Design review of the part built by this model. Coordinates are the model's own, in mm. Give positions to 0.01 mm unless a question says otherwise; leave off trailing zeros. Order: outer loops, then holes, each group sorted by start corner. A loop starts at its lowest first (then second) coordinate and runs counter-clockwise, first axis right, second up. Notation, with made-up numbers: (40, 6) -> (68, 6) arc R34 ccw to (68, 36) -> close; hole circle Ø5 at (74, 82.5). An arc over 180 degrees is marked (long way). Return JSON: item names as keys, results as strings.
```python
from build123d import *

# Parameters (mm, degrees)
SKETCH1_W           = 93
SKETCH1_H           = 102.7
BOSS_EXTRUDE2_DEPTH = 6
SKETCH3_W           = 35
SKETCH3_H           = 100
BOSS_EXTRUDE3_DEPTH = 2.5
SKETCH4_W           = 8.5
SKETCH4_H           = 15
BOSS_EXTRUDE4_DEPTH = 24
SKETCH5_R           = 2
CUT_EXTRUDE1_DEPTH  = 50
SKETCH6_R           = 8.115
CUT_EXTRUDE2_DEPTH  = 50
SKETCH7_R           = 11
CUT_EXTRUDE3_DEPTH  = 50
EXTRUDE_THIN1_START = -3.5
SKETCH7_AGAIN_R     = 11
SKETCH7_AGAIN_R_2   = 9
EXTRUDE_THIN1_DEPTH = 2.5
EXTRUDE_THIN2_START = -3.5
SKETCH6_2_R         = 8.115
SKETCH6_2_R_2       = 6.115
EXTRUDE_THIN2_DEPTH = 5


with BuildPart() as part:
    # Sketch1 → Boss-Extrude2 (new body)
    with BuildSketch(Plane.XY):
        with Locations((-29.68705036, 16.278057554)):
            Rectangle(SKETCH1_W, SKETCH1_H)
    extrude(amount=BOSS_EXTRUDE2_DEPTH)

    # Sketch3 → Boss-Extrude3 (add)
    with BuildSketch(Plane(origin=(0, 0, 0), x_dir=(-1, 0, 0), z_dir=(0, 0, -1))):
        with Locations((0.68705036, 14.928057554)):
            Rectangle(SKETCH3_W, SKETCH3_H)
    extrude(amount=BOSS_EXTRUDE3_DEPTH)

    # Sketch4 → Boss-Extrude4 (add)
    with BuildSketch(Plane(origin=(16.81294964, 0, 0), x_dir=(0, 0, -1), z_dir=(1, 0, 0))):
        with Locations((-1.75, -12.571942446)):
            Rectangle(SKETCH4_W, SKETCH4_H)
    extrude(amount=BOSS_EXTRUDE4_DEPTH)

    # Sketch5 → Cut-Extrude1 (cut)
    with BuildSketch(Plane(origin=(0, -5.071942446, 0), x_dir=(1, 0, 0), z_dir=(0, 1, 0))):
        with Locations(Location((28.81294964, -0.5, 0), (0, 0, 180))):
            Circle(SKETCH5_R)
    extrude(amount=-CUT_EXTRUDE1_DEPTH, mode=Mode.SUBTRACT)

    # Sketch6 → Cut-Extrude2 (cut)
    with BuildSketch(Plane(origin=(0, 0, -2.5), x_dir=(-1, 0, 0), z_dir=(0, 0, -1))):
        with Locations((-1.81294964, -24.571942446)):
            Circle(SKETCH6_R)
    extrude(amount=-CUT_EXTRUDE2_DEPTH, mode=Mode.SUBTRACT)

    # Sketch7 → Cut-Extrude3 (cut)
    with BuildSketch(Plane(origin=(0, 0, 0), x_dir=(-1, 0, 0), z_dir=(0, 0, -1))):
        with Locations((53.18705036, 36.928057554)):
            Circle(SKETCH7_R)
    extrude(amount=-CUT_EXTRUDE3_DEPTH, mode=Mode.SUBTRACT)

    # Sketch7 again → Extrude-Thin1 (add)
    with BuildSketch(Plane(origin=(0, 0, 0), x_dir=(-1, 0, 0), z_dir=(0, 0, -1)).offset(EXTRUDE_THIN1_START)):
        with Locations((53.18705036, 36.928057554)):
            Circle(SKETCH7_AGAIN_R)
        with Locations((53.18705036, 36.928057554)):
            Circle(SKETCH7_AGAIN_R_2, mode=Mode.SUBTRACT)
    extrude(amount=-EXTRUDE_THIN1_DEPTH)

    # Sketch6<2> → Extrude-Thin2 (add)
    with BuildSketch(Plane(origin=(0, 0, -2.5), x_dir=(-1, 0, 0), z_dir=(0, 0, -1)).offset(EXTRUDE_THIN2_START)):
        with Locations((-1.81294964, -24.571942446)):
            Circle(SKETCH6_2_R)
        with Locations((-1.81294964, -24.571942446)):
            Circle(SKETCH6_2_R_2, mode=Mode.SUBTRACT)
    extrude(amount=-EXTRUDE_THIN2_DEPTH)


solid = part.part
```
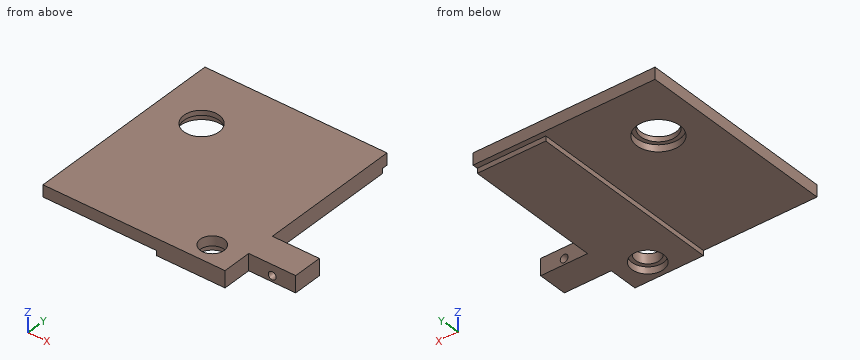
Item 1: Add section D-D (z = 4.75). Give the boundary of the cut face in (x, y) (3 decimals).
Result set:
{"outline": "(-76.187, -35.072) -> (16.813, -35.072) -> (16.813, -20.072) -> (40.813, -20.072) -> (40.813, -5.072) -> (16.813, -5.072) -> (16.813, 67.628) -> (-76.187, 67.628) -> close; hole circle Ø18 at (-53.187, 36.928); hole circle Ø12.23 at (1.813, -24.572)"}
Item 2: Add section C-C (y = 59). Give the boundary of the cut face in (x, z).
Result set:
{"outline": "(-76.19, 0) -> (-18.19, 0) -> (-18.19, -2.5) -> (16.81, -2.5) -> (16.81, 6) -> (-76.19, 6) -> close"}
Item 3: Add section A-A (y = 41). Give the boundary of the cut face in (x, z).
Result set:
{"outline": "(-76.19, 0) -> (-63.41, 0) -> (-63.41, 3.5) -> (-61.21, 3.5) -> (-61.21, 6) -> (-76.19, 6) -> close; (-45.16, 3.5) -> (-42.97, 3.5) -> (-42.97, 0) -> (-18.19, 0) -> (-18.19, -2.5) -> (16.81, -2.5) -> (16.81, 6) -> (-45.16, 6) -> close"}
Item 4: Add section B-B (x = -3). Give the boundary of the cut face in (y, z).
Result set:
{"outline": "(-35.07, -2.5) -> (-31.11, -2.5) -> (-31.11, 1) -> (-28.34, 1) -> (-28.34, 6) -> (-35.07, 6) -> close; (-20.8, 1) -> (-18.04, 1) -> (-18.04, -2.5) -> (64.93, -2.5) -> (64.93, 0) -> (67.63, 0) -> (67.63, 6) -> (-20.8, 6) -> close"}
Item 5: Wall thickness on L1, parallel to Y at x = 33.5, z = -0.5; L2, parallel to X at y = 48, z = 4.75; L3, parallel to X at y = -30, z = 2: over which ranges is each line inside the solid? List them lowest first. Write a range as [from, to].
Result set:
{"L1": "y = [-20.07, -5.07]", "L2": "x = [-76.19, 16.81]", "L3": "x = [-76.19, -1], [4.63, 16.81]"}
Item 6: For pin 1 (11 mm diameter, centred on x = -53.19, y = 36.93, fed in from +Z); pin 2 (2 mm diameter, centred on x = -3.5, z = -1.5, fed in from +Y); pin 3 (2.5 mm diameter, centred on x = 32, z = 1, fed in from +Y); pin 4 (2.5 mm diameter, centred on y = -25.5, z = 1.5, fed in from +X), all flat-tipped, find the tip position at first contact; note any pin that passes through.
Result set:
{"pin 1": "passes through", "pin 2": "stops at y = 64.93", "pin 3": "stops at y = -5.07", "pin 4": "stops at x = 16.81"}
